from build123d import *
from build123d.topology import SkipClean

# Parameters (mm, degrees)
BOSS_EXTRUDE1_DEPTH      = 4
SKETCH4_R                = 8
BOSS_EXTRUDE2_DEPTH      = 2
BOSS_EXTRUDE3_DEPTH      = 3
F_3_0_3_DIAMETER_HOLE1_D = 3
F_6_0_6_DIAMETER_HOLE1_D = 6
BOSS_EXTRUDE4_START      = 2
SKETCH12_R               = 3
SKETCH12_R_2             = 2
BOSS_EXTRUDE4_DEPTH      = 2


with BuildPart() as part:
    # Sketch1 → Boss-Extrude1 (new body)
    with BuildSketch(Plane.XY):
        with BuildLine():
            Line((3.123869731, 7.364878676), (12, 3.6))
            Line((12, 3.6), (23.9, 3.6))
            ThreePointArc((23.9, 3.6), (27.5, 0), (23.9, -3.6))
            Line((23.9, -3.6), (12, -3.6))
            Line((12, -3.6), (3.123869731, -7.364878676))
            ThreePointArc((3.123869731, -7.364878676), (-8, 0), (3.123869731, 7.364878676))
        make_face()
    extrude(amount=BOSS_EXTRUDE1_DEPTH)

    # Sketch4 → Boss-Extrude2 (add)
    with SkipClean():  # the faces are left unmerged after this step: merging them gives an invalid solid
        with BuildSketch(Plane.XY.offset(4)):
            with Locations(Location((0, 0, 0), (0, 0, 67.015399011))):
                Circle(SKETCH4_R)
        extrude(amount=BOSS_EXTRUDE2_DEPTH)

    # Sketch5 → Boss-Extrude3 (add)
    with SkipClean():  # the faces are left unmerged after this step: merging them gives an invalid solid
        with BuildSketch(Plane.XY.offset(4)):
            with BuildLine():
                Line((23.9, -2.5), (19.9, -2.5))
                ThreePointArc((19.9, -2.5), (17.4, 0), (19.9, 2.5))
                Line((19.9, 2.5), (23.9, 2.5))
                ThreePointArc((23.9, 2.5), (26.4, 0), (23.9, -2.5))
            make_face()
        extrude(amount=BOSS_EXTRUDE3_DEPTH)

    # Ø3.0 (3) Diameter Hole1 (through all)
    with Locations(Plane(origin=(0, 0, 0), x_dir=(-1, 0, 0), z_dir=(0, 0, -1))):
        with Locations((-23.9, 0), (-19.9, 0)):
            Hole(F_3_0_3_DIAMETER_HOLE1_D / 2)

    # Ø6.0 (6) Diameter Hole1 (through all)
    with Locations(Plane(origin=(0, 0, 0), x_dir=(-1, 0, 0), z_dir=(0, 0, -1))):
        with Locations((0, 0)):
            Hole(F_6_0_6_DIAMETER_HOLE1_D / 2)

    # Sketch12 → Boss-Extrude4 (add)
    with SkipClean():  # the faces are left unmerged after this step: merging them gives an invalid solid
        with BuildSketch(Plane.XY.offset(BOSS_EXTRUDE4_START)):
            Circle(SKETCH12_R)
            with Locations(Location((0, 0, 0), (0, 0, 180))):
                Circle(SKETCH12_R_2, mode=Mode.SUBTRACT)
        extrude(amount=-BOSS_EXTRUDE4_DEPTH)


solid = part.part
Design review of the part built by this model. Coordinates are the model's own, in mm. A direction names the side the tool comes from. Round coordinates to 2 decimals unless told otherwise and drop trailing zeros. Write each loop counter-clockwise with the first axis right and the second up, starting at its lowest first coordinate (ties: lowest second). Pieces come first, ordered by that corner, then holes.
Item 1: Draft analysis for pull direction Y (two halves, no side actions). For faces 6 (the flat face through (18, -3.6, 2)), 7 (the cylindrical face through (0, 2, 1)), 8 (the flat face through (18, 3.6, 2)), state which applies: released by +Y, released by -Y, zero draft, split by the parting line, or undercut.
Item 2: Wall thickness on L1, parallel to Y at x = 0, z = 5; L2, parallel to Y at x = 19.9, z = 2.25; L3, parallel to Z at x = -3, y = -5.75: over which ranges is each line inside the solid? List them lowest first.
Item 3: Consider section B-B on z = 5.25. Give the boundary of the cut face in (x, y), and give its area (3 significant figures).
Item 4: Consider section A-A on y = 0. Give the boundary of the cut face in (x, z).
Item 5: For faces 1 (the flat face through (22, 2.5, 5)), 2 (the cylindrical face through (26.4, 0.1, 5.5)), 3 (the flat face through (1, 3, 6)), 4 (the flat face through (22, -2.5, 5)), 5 (the cylindrical face through (17.4, -0.1, 5.5)), list the 3-axis set-ups (+Z, -Z, +X, -X, +Y, -Y) from which the entire face can be reached by the end or side of a thin tool; tool diameter is ignored.
Item 6: Consider section D-D on z = 1.5. Give the boundary of the cut face in (x, y).
Item 7: For pin 1 Ø3 at (x, y) = (-1, -1.5) entering from +Z; pin 2 Ø0.9 at (x, z) = (22.5, 5) entering from -Y; pin 3 Ø4 at (x, y) = (13, -1) entering from +Z, all flat-tipped, find the tip position at first contact; note any pin that passes through.
Item 8: Consider section C-C on x = 0. Give the boundary of the cut face in (y, z).
Check values:
1. face 6: released by -Y
1. face 7: undercut
1. face 8: released by +Y
2. L1: y = -8 to -3, 3 to 8
2. L2: y = -3.6 to -1.5, 1.5 to 3.6
2. L3: z = 0 to 6
3. outline: circle Ø16 at (0, 0); (19.9, -2.5) - (23.9, -2.5) arc R2.5 ccw to (23.9, 2.5) - (19.9, 2.5) arc R2.5 ccw to start; hole circle Ø6 at (0, 0); hole circle Ø3 at (19.9, 0); hole circle Ø3 at (23.9, 0)
3. area: 198 mm2
4. outline: (-8, 0) - (-2, 0) - (-2, 2) - (-3, 2) - (-3, 6) - (-8, 6) - close; (2, 0) - (18.4, 0) - (18.4, 7) - (17.4, 7) - (17.4, 4) - (8, 4) - (8, 6) - (3, 6) - (3, 2) - (2, 2) - close; (21.4, 0) - (22.4, 0) - (22.4, 7) - (21.4, 7) - close; (25.4, 0) - (27.5, 0) - (27.5, 4) - (26.4, 4) - (26.4, 7) - (25.4, 7) - close
5. face 1: +Z, +X, +Y
5. face 2: +Z, +X
5. face 3: +Z, -X, +Y, -Y
5. face 4: +Z, +X, -Y
5. face 5: +Z
6. outline: (3.12, -7.36) - (12, -3.6) - (23.9, -3.6) arc R3.6 ccw to (23.9, 3.6) - (12, 3.6) - (3.12, 7.36) arc R8 ccw (long way) to start; hole circle Ø4 at (0, 0); hole circle Ø3 at (19.9, 0); hole circle Ø3 at (23.9, 0)
7. pin 1: stops at z = 6
7. pin 2: stops at y = -2.5
7. pin 3: stops at z = 4
8. outline: (-8, 0) - (-2, 0) - (-2, 2) - (-3, 2) - (-3, 6) - (-8, 6) - close; (2, 0) - (8, 0) - (8, 6) - (3, 6) - (3, 2) - (2, 2) - close
